from build123d import *

# Parameters (mm, degrees)
MODEL_R         = 3.5
MODEL_R_2       = 0.7
EXTRUDE_1_DEPTH = 0.5
EXTRUDE2_DEPTH  = 0.1


with BuildPart() as part:
    # Model → Бобышка-Вытянуть1 (new, symmetric)
    with BuildSketch(Plane.XY):
        with BuildLine():
            Line((-3.5, 7), (-2.039607805, 7))
            ThreePointArc((-2.039607805, 7), (-1.731001106, 7.106602104), (-1.553986899, 7.380952381))
            ThreePointArc((-1.553986899, 7.380952381), (0, 8.6), (1.553986899, 7.380952381))
            ThreePointArc((1.553986899, 7.380952381), (1.731001106, 7.106602104), (2.039607805, 7))
            Line((2.039607805, 7), (3.5, 7))
            ThreePointArc((3.5, 7), (3.853553391, 6.853553391), (4, 6.5))
            Line((4, 6.5), (4, 6))
            ThreePointArc((4, 6), (4.146446609, 5.646446609), (4.5, 5.5))
            Line((4.5, 5.5), (6.6, 5.5))
            ThreePointArc((6.6, 5.5), (6.953553391, 5.353553391), (7.1, 5))
            Line((7.1, 5), (7.1, -5))
            ThreePointArc((7.1, -5), (6.953553391, -5.353553391), (6.6, -5.5))
            Line((6.6, -5.5), (4.5, -5.5))
            ThreePointArc((4.5, -5.5), (4.146446609, -5.646446609), (4, -6))
            Line((4, -6), (4, -6.5))
            ThreePointArc((4, -6.5), (3.853553391, -6.853553391), (3.5, -7))
            Line((3.5, -7), (2.039607805, -7))
            ThreePointArc((2.039607805, -7), (1.731001106, -7.106602104), (1.553986899, -7.380952381))
            ThreePointArc((1.553986899, -7.380952381), (0, -8.6), (-1.553986899, -7.380952381))
            ThreePointArc((-1.553986899, -7.380952381), (-1.731001106, -7.106602104), (-2.039607805, -7))
            Line((-2.039607805, -7), (-3.5, -7))
            ThreePointArc((-3.5, -7), (-3.853553391, -6.853553391), (-4, -6.5))
            Line((-4, -6.5), (-4, -6))
            ThreePointArc((-4, -6), (-4.146446609, -5.646446609), (-4.5, -5.5))
            Line((-4.5, -5.5), (-8.2, -5.5))
            ThreePointArc((-8.2, -5.5), (-8.553553391, -5.353553391), (-8.7, -5))
            Line((-8.7, -5), (-8.7, 5))
            ThreePointArc((-8.7, 5), (-8.553553391, 5.353553391), (-8.2, 5.5))
            Line((-8.2, 5.5), (-4.5, 5.5))
            ThreePointArc((-4.5, 5.5), (-4.146446609, 5.646446609), (-4, 6))
            Line((-4, 6), (-4, 6.5))
            ThreePointArc((-4, 6.5), (-3.853553391, 6.853553391), (-3.5, 7))
        make_face()
        Circle(MODEL_R, mode=Mode.SUBTRACT)
        with Locations((0, 7)):
            Circle(MODEL_R_2, mode=Mode.SUBTRACT)
        with Locations((0, -7)):
            Circle(MODEL_R_2, mode=Mode.SUBTRACT)
    extrude(amount=EXTRUDE_1_DEPTH, both=True)

    # Sketch2 → Extrude2 (cut)
    with BuildSketch(Plane.XY.offset(0.5)):
        Polygon((-9.557418436, -3.8), (-4.9, -3.8), (-4.9, 3.8), (-9.557418436, 3.8), (-9.557418436, 3.4), (-5.3, 3.4), (-5.3, 1.462476295), (-9.557418436, 1.462476295), (-9.557418436, 1.062476295), (-5.3, 1.062476295), (-5.3, -1.062476295), (-9.557418436, -1.062476295), (-9.557418436, -1.462476295), (-5.3, -1.462476295), (-5.3, -3.4), (-9.557418436, -3.4), align=None)
        Polygon((7.739654587, -1.8), (7.739654587, -1.4), (4.3, -1.4), (4.3, 1.4), (7.739654587, 1.4), (7.739654587, 1.8), (3.9, 1.8), (3.9, -1.8), align=None)
    extrude(amount=-EXTRUDE2_DEPTH, mode=Mode.SUBTRACT)


solid = part.part
Check sheet for the modelled part. Datum: model origin and axes. Units: mm. A direction names the side the tool comes from. Give positions to 0.01 mm unless a question says otherwise; leave off trailing zeros. Order: outer loops, then holes, each group sorted by start corner. A loop starts at its lowest first (then second) coordinate and runs counter-clockwise, first axis right, second up. Notation, with made-up numbers: (77, -32) - (121, -32) arc R21 ccw to (121, 6) - close; hole circle Ø8 at (-34.5, 25). An arc over 180 degrees is marked (long way). Answer as CSV lines item,"result".
1. Section check A-A (x = 0). Record the boundary of the cut face in (y, z).
Result sheet:
outline,"(-8.6, -0.5) - (-7.7, -0.5) - (-7.7, 0.5) - (-8.6, 0.5) - close; (-6.3, -0.5) - (-3.5, -0.5) - (-3.5, 0.5) - (-6.3, 0.5) - close; (3.5, -0.5) - (6.3, -0.5) - (6.3, 0.5) - (3.5, 0.5) - close; (7.7, -0.5) - (8.6, -0.5) - (8.6, 0.5) - (7.7, 0.5) - close"
2. Tool access check on faces 1 (the face through (6, 5.5, 0)), 2 (the face through (-6, -5.5, 0)), 3 (the face through (6, -5.5, 0)). Record the directions out of +Z, -Z, +X, -X, +Y, -Y that give a thin tool (end or side, any length) a straight path to the whole face; none if there is none.
Result sheet:
face 1,"+Z, -Z, +X, +Y"
face 2,"+Z, -Z, -X, -Y"
face 3,"+Z, -Z, +X, -Y"
3. Section check C-C (x = -5.5). Record the boundary of the cut face in (y, z).
Result sheet:
outline,"(-5.5, -0.5) - (5.5, -0.5) - (5.5, 0.5) - (3.8, 0.5) - (3.8, 0.4) - (3.4, 0.4) - (3.4, 0.5) - (1.46, 0.5) - (1.46, 0.4) - (1.06, 0.4) - (1.06, 0.5) - (-1.06, 0.5) - (-1.06, 0.4) - (-1.46, 0.4) - (-1.46, 0.5) - (-3.4, 0.5) - (-3.4, 0.4) - (-3.8, 0.4) - (-3.8, 0.5) - (-5.5, 0.5) - close"
4. Section check D-D (z = 0). State how many separate pieces and enclosed holes the cut face has, then the cut area to 3 significant figures.
Result sheet:
separate pieces,"1"
enclosed holes,"3"
area,"164 mm²"
5. Scan lines: probe 1 along Y at (x, z) = (0, -0.3); probe 2 along X at (y, z) = (-0.25, 0.45); probe 3 along Y at (x, z) = (3, 0.05). Record each from-to range of solid material in increasing order. Write a range as from..to.
Result sheet:
probe 1,"-8.6..-7.7, -6.3..-3.5, 3.5..6.3, 7.7..8.6"
probe 2,"-8.7..-5.3, -4.9..-3.49, 3.49..3.9, 4.3..7.1"
probe 3,"-7..-1.8, 1.8..7"
6. Section check B-B (y = 0). Record the boundary of the cut face in (x, z).
Result sheet:
outline,"(-8.7, -0.5) - (-3.5, -0.5) - (-3.5, 0.5) - (-4.9, 0.5) - (-4.9, 0.4) - (-5.3, 0.4) - (-5.3, 0.5) - (-8.7, 0.5) - close; (3.5, -0.5) - (7.1, -0.5) - (7.1, 0.5) - (4.3, 0.5) - (4.3, 0.4) - (3.9, 0.4) - (3.9, 0.5) - (3.5, 0.5) - close"
7. Go/stop test with a flat-tipped pin: P1, Ø0.6, axis at y = 6.5, z = 0, coming from the +X side. Record where the tip stops, or that it passes through.
Result sheet:
P1,"x = 4"
8. Mould release check, pull along X, two halves, no side actions. Record for faces 4 (the face through (0, -8.6, 0)), 5 (the face through (0.38, -6.41, -0.01)), 6 (the face through (-6, 5.5, 0)): released by +X, released by -X, zero draft, split by the parting line, or undercut.
Result sheet:
face 4,"split by the parting line"
face 5,"undercut"
face 6,"zero draft"
